```python
from build123d import *

# Parameters (mm, degrees)
FILLET1_R = 1


with BuildPart() as part:
    # Sketch1 → Revolve1 (revolve)
    with BuildSketch(Plane(origin=(0, 0, 0), x_dir=(0, 0, -1), z_dir=(1, 0, 0))):
        Polygon((7.5, 17.5), (9, 17.5), (9, 1.75), (11, 1.75), (11, -17.5), (9.5, -17.5), (9.5, -1.75), (7.5, -1.75), align=None)
    revolve(axis=Axis((0, -17.5, 0), (0, 1, 0)))

    # Fillet1
    fillet1_edges = [part.edges().sort_by_distance(p)[0] for p in [
        (0, 1.75, 11),
        (0, 1.75, 9),
    ]]
    fillet(fillet1_edges, radius=FILLET1_R - 0.0001)  # a hair under: the kernel refuses the full size


solid = part.part
```
Could you check a few things on this model? Use its own coordinates, in mm. A direction names the side the tool comes from. Round coordinates to 2 decimals unless told otherwise and drop trailing zeros. Loops run counter-clockwise (first coordinate to the right, second up) from the corner with the lowest first, then second, coordinate; pieces in that order, holes last.
Q1. Please list where these lines run through material, in increasing order: L1, parallel to X at y = 13.25, z = 0; L2, parallel to Z at x = 0, y = -8.5.
Q2. I want a section at C-C (y = -10). Write out the boundary of the cut face in (x, z).
Q3. For P1, Ø1.5, axis at y = -12.5, z = -4.5, coming from the -X side; P2, Ø1.5, axis at y = -11, z = -1, coming from the -X side; P3, Ø4, axis at x = -5, y = 11.5, coming from the -Z side, each with a flat end and sliding along its axis, tell me the tip position at first contact or that it passes through.
Q4. Thinking about a two-plate mould opening in Z: for faces 3 (the cylindrical face through (10.74, -8.5, 2.38)), 4 (the cylindrical face through (8.43, -9.51, -4.38)), 5 (the flat face through (-8, -1.75, -1)), 6 (the flat face through (-7.4, 17.5, -2)), which applies, pulls with the +Z half, pulls with the -Z half, needs draft (parallel to the pull), parting line crosses it, or undercut?
Q5. I want a section at D-D (y = 6). Write out the boundary of the cut face in (x, z).
Q6. On a 3-axis mill with a long thin cutter (end or side, diameter ignored), from which of +Z, -Z, +X, -X, +Y, -Y can I reach the whole of each face in a straight line? I mean faces 1 (the cylindrical face through (-8.923, 10.022, 1.172)), 2 (the flat face through (0, -17.5, 10)). Say none if no direction works.
Answer below:
1. L1: x = -9 to -7.5, 7.5 to 9
1. L2: z = -11 to -9.5, 9.5 to 11
2. outline: circle Ø22 at (0, 0); hole circle Ø19 at (0, 0)
3. P1: stops at x = -10.34
3. P2: stops at x = -11
3. P3: stops at z = -8.49
4. face 3: parting line crosses it
4. face 4: undercut
4. face 5: undercut
4. face 6: needs draft
5. outline: circle Ø18 at (0, 0); hole circle Ø15 at (0, 0)
6. face 1: +Y
6. face 2: +Z, -Z, +X, -X, -Y
